```python
from build123d import *

# Parameters (mm, degrees)
SKETCH_1_R             = 6.25
SM_BASE_FLANGE_1_DEPTH = 4


# Sheet-metal steps are written as plain solids
with BuildPart() as part:
    # Sketch 1 → Базовая кромка1 (new body)
    with BuildSketch(Plane(origin=(0, 0, 0), x_dir=(1, 0, 0), z_dir=(0, 1, 0))):
        with BuildLine():
            Line((12, 15), (-12, 15))
            ThreePointArc((-12, 15), (-14.121320344, 14.121320344), (-15, 12))
            Line((-15, 12), (-15, -12))
            ThreePointArc((-15, -12), (-14.121320344, -14.121320344), (-12, -15))
            Line((-12, -15), (12, -15))
            ThreePointArc((12, -15), (14.121320344, -14.121320344), (15, -12))
            Line((15, -12), (15, 12))
            ThreePointArc((15, 12), (14.121320344, 14.121320344), (12, 15))
        make_face()
        with Locations(Location((0, 0, 0), (0, 0, 270))):
            Circle(SKETCH_1_R, mode=Mode.SUBTRACT)
    extrude(amount=-SM_BASE_FLANGE_1_DEPTH)


solid = part.part
```
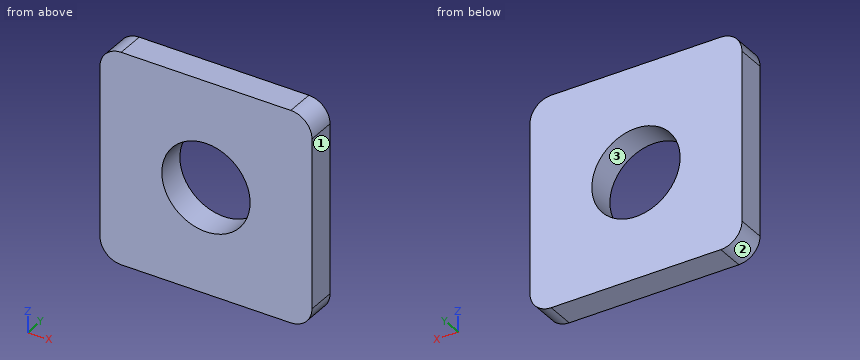
Geometry check sheet. Reference: the model listing, model coordinates, mm. Face numbers are marked on the shaded views. Coordinates: 2 decimals unless noted, no trailing zeros. Write each loop counter-clockwise with the first axis right and the second up, starting at its lowest first coordinate (ties: lowest second). Pieces come first, ordered by that corner, then holes. Notation, with made-up numbers: M 24,25 L 79,25 A16 ccw 79,56 Z; hole C -23.75,65.5 d6. An arc over 180 degrees is marked long. One line per item, written item: value. Start each with the question number.
(1) Sectioned sample at D-D, the plane z = 13.25. Enter the section's corners in (x, y), and give its area (3 significant figures).
(2) Sectioned sample at A-A, the plane z = 0. Enter the section's corners in (x, y), and give its area (3 significant figures).
(3) Sectioned sample at B-B, the plane x = 0. Enter the section's corners in (y, z), and give its area (3 significant figures).
(4) Scan lines: line 1 along X through (y, z) = (-1.3, 0); line 2 along X through (y, z) = (-1.55, -3.5); line 3 along Z through (x, y) = (0.5, -2). Record each from-to range of solid material in increasing order. Write a range as [from, to].
(5) Sectioned sample at C-C, the plane y = -2.8. Enter the section's corners in (x, z).
(6) Release check for a two-part mould opening along Z. For the marked faces 1, 2 and 3 record: released by +Z, released by -Z, zero draft, split by the parting line, or undercut.
Filled sheet:
1. outline: M -14.73,-4 L 14.73,-4 L 14.73,0 L -14.73,0 Z
1. area: 118 mm²
2. outline: M -15,-4 L -6.25,-4 L -6.25,0 L -15,0 Z; M 6.25,-4 L 15,-4 L 15,0 L 6.25,0 Z
2. area: 70.0 mm²
3. outline: M -4,-15 L 0,-15 L 0,-6.25 L -4,-6.25 Z; M -4,6.25 L 0,6.25 L 0,15 L -4,15 Z
3. area: 70.0 mm²
4. line 1: [-15, -6.25], [6.25, 15]
4. line 2: [-15, -5.18], [5.18, 15]
4. line 3: [-15, -6.23], [6.23, 15]
5. outline: M -15,-12 A3 ccw -12,-15 L 12,-15 A3 ccw 15,-12 L 15,12 A3 ccw 12,15 L -12,15 A3 ccw -15,12 Z; hole C 0,0 d12.5
6. face 1: zero draft
6. face 2: released by -Z
6. face 3: undercut
